Verification items for the finished model (mm, model axes). Face numbers are marked on the shaded views. A direction names the side the tool comes from. Coordinates: 2 decimals unless noted, no trailing zeros. Order: outer loops, then holes, each group sorted by start corner. A loop starts at its lowest first (then second) coordinate and runs counter-clockwise, first axis right, second up. Notation, with made-up numbers: M 9.25,19 L 33.25,19 A32 cw 33.25,53 Z; hole C 53.25,42 d1. An arc over 180 degrees is marked long. Use one line per item in the form item = value. Start each with the question number.
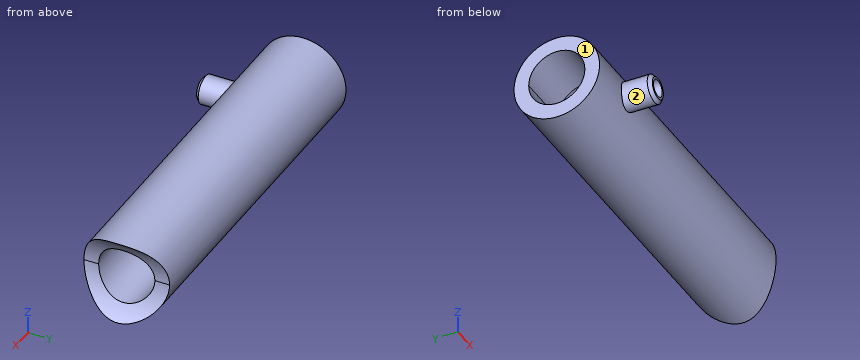
```python
from build123d import *
from build123d import SkipClean  # not in build123d's __all__

# Parameters (mm, degrees)
F0_R      = 12.5
F0_R_2    = 7.5
F1_DEPTH  = 64
F2_R      = 38.1
F2_R_2    = 25
F3_DEPTH  = 100
F4_DEPTH  = 50
F5_SIZE   = 3
F6_R      = 25
F7_DEPTH  = 200
F8_R      = 7.5
F9_DEPTH  = 50
F10_DEPTH = 100
F11_R     = 7.5
F12_DEPTH = 50
F13_DEPTH = 75


with BuildPart() as f1:
    # F0 (on Front) → F1 (new body)
    with BuildSketch(Plane.XZ):
        Circle(F0_R)
        Circle(F0_R_2, mode=Mode.SUBTRACT)
    extrude(amount=F1_DEPTH)

    # F2 (on Right) → F3 (join)
    with BuildSketch(Plane.YZ):
        Circle(F2_R)
        Circle(F2_R_2, mode=Mode.SUBTRACT)
    extrude(amount=F3_DEPTH)

    # F2 (on Right) → F4 (join)
    with BuildSketch(Plane.YZ):
        Circle(F2_R)
        Circle(F2_R_2, mode=Mode.SUBTRACT)
    extrude(amount=-F4_DEPTH)

    # F5
    f5_edges = [f1.edges().sort_by_distance(p)[0] for p in [
        (-12.5, -64, 0),
    ]]
    chamfer(f5_edges, length=F5_SIZE)

    # F6 (on face) → F7 (cut)
    with BuildSketch(Plane(origin=(-50, 0, 0), x_dir=(0, -1, 0), z_dir=(-1, 0, 0))):
        Circle(F6_R)
    extrude(amount=-F7_DEPTH, mode=Mode.SUBTRACT)

    # F8 (on face) → F9 (cut)
    with BuildSketch(Plane.XZ.offset(64)):
        Circle(F8_R)
    extrude(amount=-F9_DEPTH, mode=Mode.SUBTRACT)

    # F10 (add): a face of the model
    f10_faces = [f1.faces().sort_by_distance(p)[0] for p in [
        (100, -37.0223692655, 0),
    ]]
    with SkipClean():  # cleaning this boolean's faces spoils the solid; the shape is the same uncleaned
        extrude(f10_faces, amount=F10_DEPTH)

    # F11 (on face) → F12 (cut)
    with BuildSketch(Plane.XZ.offset(64)):
        Circle(F11_R)
    with SkipClean():  # cleaning this boolean's faces spoils the solid; the shape is the same uncleaned
        extrude(amount=-F12_DEPTH, mode=Mode.SUBTRACT)

    # F13 (add): a face of the model
    f13_faces = [f1.faces().sort_by_distance(p)[0] for p in [
        (200, -37.0223692655, 0),
    ]]
    extrude(f13_faces, amount=F13_DEPTH)

    # F14 (on Top) → F15 (revolve, cut)
    with BuildSketch(Plane.XY):
        Polygon((280.1408666709, 52.4849742776), (252.6145875454, 51.9348941743), (252.6145875454, -50.6588555872), (280.1408666709, -51.4342445287), align=None)
    with SkipClean():  # cleaning this boolean's faces spoils the solid; the shape is the same uncleaned
        revolve(axis=Axis((303.6976158619, 0.4289562068, 0), (0, -1, 0)), mode=Mode.SUBTRACT)


solid = f1.part
```
1. Cross-section at D-D on z = -3. Give the number of separate pieces and of enclosed holes in the cut face, and give its area (3 significant figures).
2. Cross-section at B-B on z = -16. Enter the section's corners in (x, y), and give its area (3 significant figures).
3. Depth check by flat-ended pin: P1, Ø3, axis at y = 27.5, z = -14.5, coming from the +X side (3 decimals); P2, Ø10, axis at y = -19, z = 28, coming from the +X side; P3, Ø6, axis at x = 163.5, y = -17.5, coming from the -Z side. Enter the tip coordinate at first touch or a pass-through.
4. Material ranges on line 1 along X through (y, z) = (-28, 0); line 2 along Y through (x, z) = (83.5, -1.5); line 3 along Z through (x, y) = (130, 0), recorded low to high.
5. Cross-section at A-A on y = 0. Enter the section's corners in (x, z).
6. Cross-section at C-C on x = 89.5. Enter the section's corners in (y, z), and give its area (3 significant figures).
7. Tool access check on the marked faces 1 and 2. Record the directions out of +Z, -Z, +X, -X, +Y, -Y that give a thin tool (end or side, any length) a straight path to the whole face; none if there is none.
Final values:
q1.separate_pieces = 3
q1.enclosed_holes = 0
q1.area = 8,050 mm2
q2.outline = M -50,-34.58 L 255.18,-34.58 L 255.18,-19.21 L -50,-19.21 Z; M -50,19.21 L 255.18,19.21 L 255.18,34.58 L -50,34.58 Z
q2.area = 9,380 mm2
q3.P1 = 255.185
q3.P2 = 264.7
q3.P3 = -35.23
q4.line_1 = -50 to -7.5, 7.5 to 252.61
q4.line_2 = -38.07 to -24.95, 24.95 to 38.07
q4.line_3 = -38.1 to -25, 25 to 38.1
q5.outline = M -50,-38.1 L 269.67,-38.1 A51.08 cw 259.15,-25 L -50,-25 Z; M -50,25 L 259.15,25 A51.08 cw 269.67,38.1 L -50,38.1 Z
q6.outline = C 0,0 d76.2; hole C 0,0 d50
q6.area = 2,600 mm2
q7.face_1 = +Z, -Z, -X, +Y, -Y
q7.face_2 = -Y
